```python
from build123d import *

# Parameters (mm, degrees)
F2_R = 12.7
F3_T = -3.175


with BuildPart() as f1:
    # F0 (on Front) → F1 (revolve)
    with BuildSketch(Plane.XZ):
        Polygon((0, 825.5), (0, 0), (533.4, 0), (533.4, 317.5), align=None)
    revolve(axis=Axis((0, 0, 412.75), (0, 0, 1)))

    # F2
    f2_edges = [f1.edges().sort_by_distance(p)[0] for p in [
        (-533.4, 0, 317.5),
    ]]
    fillet(f2_edges, radius=F2_R)

    # F3
    f3_openings = [f1.faces().sort_by_distance(p)[0] for p in [
        (0, 0, 0),
    ]]
    offset(amount=F3_T, openings=f3_openings)


solid = f1.part
```
Verification items for the finished model (mm, model axes). A direction names the side the tool comes from. Coordinates: 2 decimals unless noted, no trailing zeros. Order: outer loops, then holes, each group sorted by start corner. A loop starts at its lowest first (then second) coordinate and runs counter-clockwise, first axis right, second up. Notation, with made-up numbers: (-23.75, 59) - (32.25, 59) arc R16 cw to (32.25, 73) - close; hole circle Ø11 at (16, -32). An arc over 180 degrees is marked (long way). Return JSON: item names as keys, results as strings.
(1) Section check A-A, the plane z = 94.5. Record the cut outline in (x, y) (3 decimals), and give its area (3 significant figures).
Filled sheet:
{"outline": "circle Ø1066.8 at (0, 0); hole circle Ø1060.45 at (0, 0)", "area": "10,600 mm^2"}
(2) Mould release check, pull along Y, two halves, no side actions. Record for faces 3 (the conical face through (136.18, 42.89, 685.14)), 4 (the conical face through (-31.08, -139.96, 688.96)): pulls with the +Y half, pulls with the -Y half, needs draft (parallel to the pull), parting line crosses it, or undercut.
Filled sheet:
{"face 3": "undercut", "face 4": "parting line crosses it"}
(3) Access from +Z, -Z, +X, -X, +Y, -Y to the whole of each face (thin tool, end or side, straight path). Record for faces 1 (the cylindrical face through (508.77, 160.22, 158.21)), 2 (the cylindrical face through (-69.025, 525.713, 158.213)).
Filled sheet:
{"face 1": "+Z, -Z", "face 2": "-Z"}
(4) Thickness scan on line 1 along Y through (x, z) = (0, 86) (3 decimals). Record the ranges inside material, lowest first.
Filled sheet:
{"line 1": "y = -533.4 to -530.225, 530.225 to 533.4"}
(5) Go/stop test with flat-tipped pins: pin 1 (12 mm diameter, centred on y = -35.5, z = 170.5, fed in from -X); pin 2 (1 mm diameter, centred on x = -357.5, y = 41, fed in from -Z); pin 3 (12 mm diameter, centred on x = 169.5, z = 575.5, fed in from +Y). Record where each tip stops, or that it passes through.
Filled sheet:
{"pin 1": "stops at x = -532.58", "pin 2": "stops at z = 477.93", "pin 3": "stops at y = 209.95"}
